Geometry check sheet. Reference: the model listing, model coordinates, mm. A direction names the side the tool comes from. Coordinates: 2 decimals unless noted, no trailing zeros. Write each loop counter-clockwise with the first axis right and the second up, starting at its lowest first coordinate (ties: lowest second). Pieces come first, ordered by that corner, then holes. Notation, with made-up numbers: (61.25, 41) -> (85.25, 41) arc R9 cw to (85.25, 54) -> close; hole circle Ø10 at (41.25, 41.5). An arc over 180 degrees is marked (long way). Answer in a Markdown table with one row per item. Add a question column.
Q1. Section check A-A, the plane x = 17. Record the boundary of the cut face in (y, z), and give its area (3 significant figures).
Q2. Thickness scan on line 1 (Y direction, x = -49, z = 23.95); line 2 (Y direction, x = -49, z = 0.9); line 3 (Y direction, x = -29.5, z = 7.5). Record the ranges inside material, lowest first.
Q3. Tool access check on faces 4 (the face through (88.315, 48, 14)), 5 (the face through (-49.195, 90.487, 23.732)). Record the directions out of +Z, -Z, +X, -X, +Y, -Y that give a thin tool (end or side, any length) a straight path to the whole face; none if there is none.
Q4. Section check D-D, the plane x = 60.5. Record the boundary of the cut face in (y, z).
Q5. Section check C-C, the plane z = 9.5. Record the boundary of the cut face in (x, y), and give its area (3 significant figures).
Q6. Release check for a two-part mould opening along Z. For faces 1 (the face through (11, 95, 25)), 2 (the face through (92.815, 48, 12)), 3 (the face through (-49, 6, 22.5)) record: pulls with the +Z half, pulls with the -Z half, needs draft (parallel to the pull), parting line crosses it, or undercut.
Q7. Section check B-B, the plane y = 44.5. Record the boundary of the cut face in (x, z).
Q8. Gauge pin test, flat ends, axial feed: P1, Ø6.5, axis at x = 71, y = 88, coming from the -Z side; P2, Ø1.5, axis at x = -19.5, y = 62.5, coming from the +Z side; P3, Ø0.8, axis at x = -68, y = 48, coming from the -Z side. Record the tip position at first contact, or that the pin passes through.
```python
from build123d import *

# Parameters (mm, degrees)
CROQUIS1_W              = 15
CROQUIS1_H              = 7
CROQUIS1_W_2            = 21.106040847
CROQUIS1_H_2            = 4.330702007
CROQUIS1_R              = 1.5
CROQUIS1_W_3            = 15.314275766
CROQUIS1_H_3            = 48.999512223
SALIENTE_EXTRUIR1_DEPTH = 2.5
SALIENTE_EXTRUIR2_DEPTH = 25.5
SALIENTE_EXTRUIR3_REACH = 135.996
CROQUIS3_W              = 155.129666141
CROQUIS3_H              = 2
REDONDEO1_R             = 3
REDONDEO2_R             = 3
CROQUIS6_W              = 172.033889696
CROQUIS6_H              = 4.948845102
CORTAR_EXTRUIR3_DEPTH   = 114.5
SALIENTE_EXTRUIR4_START = -2.5
CROQUIS7_W              = 6
CROQUIS7_H              = 6.5
CROQUIS7_R              = 1.5
SALIENTE_EXTRUIR4_DEPTH = 2.5


with BuildPart() as part:
    # Croquis1 → Saliente-Extruir1 (new body)
    with BuildSketch(Plane.XY):
        with BuildLine():
            Line((92.815390375, 97), (-66.814275766, 97))
            ThreePointArc((-66.814275766, 97), (-70.349809672, 95.535533906), (-71.814275766, 92))
            Line((-71.814275766, 92), (-71.814275766, 5))
            ThreePointArc((-71.814275766, 5), (-70.349809672, 1.464466094), (-66.814275766, 0))
            Line((-66.814275766, 0), (92.815390375, 0))
            Line((92.815390375, 0), (92.815390375, 97))
        make_face()
        with Locations((59.815390375, 8.5)):
            Rectangle(CROQUIS1_W, CROQUIS1_H, mode=Mode.SUBTRACT)
        with Locations((16.385259295, 89.834648996)):
            Rectangle(CROQUIS1_W_2, CROQUIS1_H_2, mode=Mode.SUBTRACT)
        with Locations((59.404912693, 88.5)):
            Rectangle(CROQUIS1_W, CROQUIS1_H, mode=Mode.SUBTRACT)
        with Locations((-49, 8)):
            Circle(CROQUIS1_R, mode=Mode.SUBTRACT)
        with Locations((-61.157137883, 48.499756112)):
            Rectangle(CROQUIS1_W_3, CROQUIS1_H_3, mode=Mode.SUBTRACT)
        with Locations((70.315390375, 8)):
            Circle(CROQUIS1_R, mode=Mode.SUBTRACT)
        with Locations((-49, 89)):
            Circle(CROQUIS1_R, mode=Mode.SUBTRACT)
        with Locations((69.850202166, 89.208902584)):
            Circle(CROQUIS1_R, mode=Mode.SUBTRACT)
    extrude(amount=SALIENTE_EXTRUIR1_DEPTH)

    # Croquis2 → Saliente-Extruir2 (add)
    with BuildSketch(Plane.XY.offset(2.5)):
        with BuildLine():
            Line((-71.814275766, 92), (-71.814275766, 5))
            ThreePointArc((-71.814275766, 5), (-70.349809672, 1.464466094), (-66.814275766, 0))
            Line((-66.814275766, 0), (92.815390375, 0))
            Line((92.815390375, 0), (92.815390375, 97))
            Line((92.815390375, 97), (-66.814275766, 97))
            ThreePointArc((-66.814275766, 97), (-70.349809672, 95.535533906), (-71.814275766, 92))
        make_face()
        with BuildLine():
            Line((-67.314275766, 92), (-67.314275766, 5))
            ThreePointArc((-67.314275766, 5), (-67.167829157, 4.646446609), (-66.814275766, 4.5))
            Line((-66.814275766, 4.5), (88.315390375, 4.5))
            Line((88.315390375, 4.5), (88.315390375, 92.5))
            Line((88.315390375, 92.5), (-66.814275766, 92.5))
            ThreePointArc((-66.814275766, 92.5), (-67.167829157, 92.353553391), (-67.314275766, 92))
        make_face(mode=Mode.SUBTRACT)
    extrude(amount=SALIENTE_EXTRUIR2_DEPTH)

    # Croquis3 → Saliente-Extruir3 (add, up to next)
    with BuildSketch(Plane(origin=(0, 4.5, 0), x_dir=(1, 0, 0), z_dir=(0, 1, 0)), mode=Mode.PRIVATE) as saliente_extruir3_sk1:
        with Locations((10.750557304, -27)):
            Rectangle(CROQUIS3_W, CROQUIS3_H)
    saliente_extruir3_tool1 = extrude(saliente_extruir3_sk1.sketch, amount=SALIENTE_EXTRUIR3_REACH, mode=Mode.PRIVATE) - part.part
    add(saliente_extruir3_tool1.solids().sort_by_distance((10.750557, 4.5, 27))[0])

    # Redondeo1
    redondeo1_edges = [part.edges().sort_by_distance(p)[0] for p in [
        (92.815390375, 97, 14),
        (92.815390375, 0, 14),
    ]]
    fillet(redondeo1_edges, radius=REDONDEO1_R)

    # Redondeo2
    redondeo2_edges = [part.edges().sort_by_distance(p)[0] for p in [
        (92.815390375, 48.5, 28),
        (11.500557304, 97, 28),
        (91.936710719, 96.121320344, 28),
        (91.936710719, 0.878679656, 28),
        (-70.349809672, 95.535533906, 28),
        (-71.814275766, 48.5, 28),
        (-70.349809672, 1.464466094, 28),
        (11.500557304, 0, 28),
    ]]
    fillet(redondeo2_edges, radius=REDONDEO2_R)

    # Croquis6 → Cortar-Extruir3 (cut)
    with BuildSketch(Plane(origin=(0, 0, 0), x_dir=(-1, 0, 0), z_dir=(0, -1, 0))):
        with Locations((-6.798445527, -27.474422551)):
            Rectangle(CROQUIS6_W, CROQUIS6_H)
    extrude(amount=-CORTAR_EXTRUIR3_DEPTH, mode=Mode.SUBTRACT)

    # Croquis7 → Saliente-Extruir4 (add)
    # profile 1 of 4: a face of its own
    with BuildSketch(Plane.XY.offset(25).offset(SALIENTE_EXTRUIR4_START)):
        with Locations((69.908799209, 89.25)):
            Rectangle(CROQUIS7_W, CROQUIS7_H)
        with Locations((69.850202166, 89.208902584)):
            Circle(CROQUIS7_R, mode=Mode.SUBTRACT)
    # profile 2 of 4: a face of its own
    with BuildSketch(Plane.XY.offset(25).offset(SALIENTE_EXTRUIR4_START)):
        with Locations((-49, 89.25)):
            Rectangle(CROQUIS7_W, CROQUIS7_H)
        with Locations((-49, 89)):
            Circle(CROQUIS7_R, mode=Mode.SUBTRACT)
    # profile 3 of 4: a face of its own
    with BuildSketch(Plane.XY.offset(25).offset(SALIENTE_EXTRUIR4_START)):
        with Locations((70.315390375, 7.75)):
            Rectangle(CROQUIS7_W, CROQUIS7_H)
        with Locations((70.315390375, 8)):
            Circle(CROQUIS7_R, mode=Mode.SUBTRACT)
    # profile 4 of 4: a face of its own
    with BuildSketch(Plane.XY.offset(25).offset(SALIENTE_EXTRUIR4_START)):
        with Locations((-49, 7.75)):
            Rectangle(CROQUIS7_W, CROQUIS7_H)
        with Locations((-49, 8)):
            Circle(CROQUIS7_R, mode=Mode.SUBTRACT)
    extrude(amount=SALIENTE_EXTRUIR4_DEPTH)


solid = part.part
```
Calculated:
| question | item | result |
|---|---|---|
| 1 | outline | (0, 0) -> (87.67, 0) -> (87.67, 2.5) -> (4.5, 2.5) -> (4.5, 25) -> (0, 25) -> close; (92, 0) -> (97, 0) -> (97, 25) -> (92.5, 25) -> (92.5, 2.5) -> (92, 2.5) -> close |
| 1 | area | 434 mm² |
| 2 | line 1 | y = 0 to 6.5, 9.5 to 11, 86 to 87.5, 90.5 to 97 |
| 2 | line 2 | y = 0 to 6.5, 9.5 to 87.5, 90.5 to 97 |
| 2 | line 3 | y = 0 to 4.5, 92.5 to 97 |
| 3 | face 4 | +Z |
| 3 | face 5 | +Z, -Z |
| 4 | outline | (0, 0) -> (5, 0) -> (5, 2.5) -> (4.5, 2.5) -> (4.5, 25) -> (0, 25) -> close; (12, 0) -> (85, 0) -> (85, 2.5) -> (12, 2.5) -> close; (92, 0) -> (97, 0) -> (97, 25) -> (92.5, 25) -> (92.5, 2.5) -> (92, 2.5) -> close |
| 5 | outline | (-71.81, 5) arc R5 ccw to (-66.81, 0) -> (89.82, 0) arc R3 ccw to (92.82, 3) -> (92.82, 94) arc R3 ccw to (89.82, 97) -> (-66.81, 97) arc R5 ccw to (-71.81, 92) -> close; hole (-67.31, 5) arc R0.5 ccw to (-66.81, 4.5) -> (88.32, 4.5) -> (88.32, 92.5) -> (-66.81, 92.5) arc R0.5 ccw to (-67.31, 92) -> close |
| 5 | area | 2,260 mm² |
| 6 | face 1 | pulls with the +Z half |
| 6 | face 2 | needs draft |
| 6 | face 3 | undercut |
| 7 | outline | (-71.81, 0) -> (-68.81, 0) -> (-68.81, 2.5) -> (-67.31, 2.5) -> (-67.31, 25) -> (-71.81, 25) -> close; (-53.5, 0) -> (92.82, 0) -> (92.82, 25) -> (88.32, 25) -> (88.32, 2.5) -> (-53.5, 2.5) -> close |
| 8 | P1 | stops at z = 0 |
| 8 | P2 | stops at z = 2.5 |
| 8 | P3 | stops at z = 2.5 |
